Design review of the part built by this model. Coordinates are the model's own, in mm. A direction names the side the tool comes from. Coordinates: 2 decimals unless noted, no trailing zeros. Order: outer loops, then holes, each group sorted by start corner. A loop starts at its lowest first (then second) coordinate and runs counter-clockwise, first axis right, second up.
from build123d import *

# Parameters (mm, degrees)
ESQUISSE1_R        = 4
BOSS_EXTRU_1_DEPTH = 6


with BuildPart() as part:
    # Esquisse1 → Boss.-Extru.1 (new body)
    with BuildSketch(Plane.XY):
        Polygon((0, 200), (0, 206), (50, 206), (50, 200), (100, 200), (100, 206), (150, 206), (150, 200), (200, 200), (200, 206), (250, 206), (250, 200), (300, 200), (300, 0), (0, 0), align=None)
        with Locations((80, 40)):
            Circle(ESQUISSE1_R, mode=Mode.SUBTRACT)
    extrude(amount=BOSS_EXTRU_1_DEPTH)


solid = part.part
1. Add section A-A (y = 40). Give the boundary of the cut face in (x, z).
2. Add section C-C (z = 1.7). Give the boundary of the cut face in (x, y).
3. Insertion check: pin 1 (3 mm diameter, centred on y = 202, z = 3, fed in from +X); pin 2 (9 mm diameter, centred on x = 80, y = 40, fed in from +Z); pin 3 (3 mm diameter, centred on x = 265, z = 3, fed in from +Y). Each pin has a flat end and moves straight along its axis. Give the tip position at first contact, or say it passes through.
4. Add section B-B (x = 80). Give the boundary of the cut face in (y, z), and give its area (3 significant figures).
5. For faces 1 (the flat face through (175, 200, 3)), 2 (the flat face through (125, 206, 3)), list the 3-axis set-ups (+Z, -Z, +X, -X, +Y, -Y) from which the entire face can be reached by the end or side of a thin tool; tool diameter is ignored.
6. To check wall thickness, follow line 1 (Y direction, x = 80, z = 2.6); line 2 (Y direction, x = 266, z = 0.45). State the ranges of each line that lie inside material, in increasing order.
7. Mouldability with a two-part tool opening along X and no side actions: class faces 3 (the flat face through (275, 200, 3)), 4 (the flat face through (200, 203, 3)), 5 (the flat face through (250, 203, 3)) as pulls with the +X half, pulls with the -X half, needs draft (parallel to the pull), parting line crosses it, or undercut.
8. Add section D-D (x = 189.5). Give the boundary of the cut face in (y, z), and give its area (3 significant figures).
Solution:
1. outline: (0, 0) - (76, 0) - (76, 6) - (0, 6) - close; (84, 0) - (300, 0) - (300, 6) - (84, 6) - close
2. outline: (0, 0) - (300, 0) - (300, 200) - (250, 200) - (250, 206) - (200, 206) - (200, 200) - (150, 200) - (150, 206) - (100, 206) - (100, 200) - (50, 200) - (50, 206) - (0, 206) - close; hole circle Ø8 at (80, 40)
3. pin 1: stops at x = 250
3. pin 2: stops at z = 6
3. pin 3: stops at y = 200
4. outline: (0, 0) - (36, 0) - (36, 6) - (0, 6) - close; (44, 0) - (200, 0) - (200, 6) - (44, 6) - close
4. area: 1,150 mm2
5. face 1: +Z, -Z, +Y
5. face 2: +Z, -Z, +X, -X, +Y
6. line 1: y = 0 to 36, 44 to 200
6. line 2: y = 0 to 200
7. face 3: needs draft
7. face 4: undercut
7. face 5: pulls with the +X half
8. outline: (0, 0) - (200, 0) - (200, 6) - (0, 6) - close
8. area: 1,200 mm2
